Could you check a few things on this drawing? It's one solid part, dimensions in mm from its lowest x, y, z. Give positions to 0.01 mm unless a question says otherwise; leave off trailing zeros. Loops run counter-clockwise (first coordinate to the right, second up) from the corner with the lowest first, then second, coordinate; pieces in that order, holes last. Notation, with made-up numbers: M -36,35.25 L 9,35.25 A30 cw 9,59.25 Z; hole C -26.75,63.25 d11. An arc over 180 degrees is marked long. Answer as a JSON object with one key per item and string values.
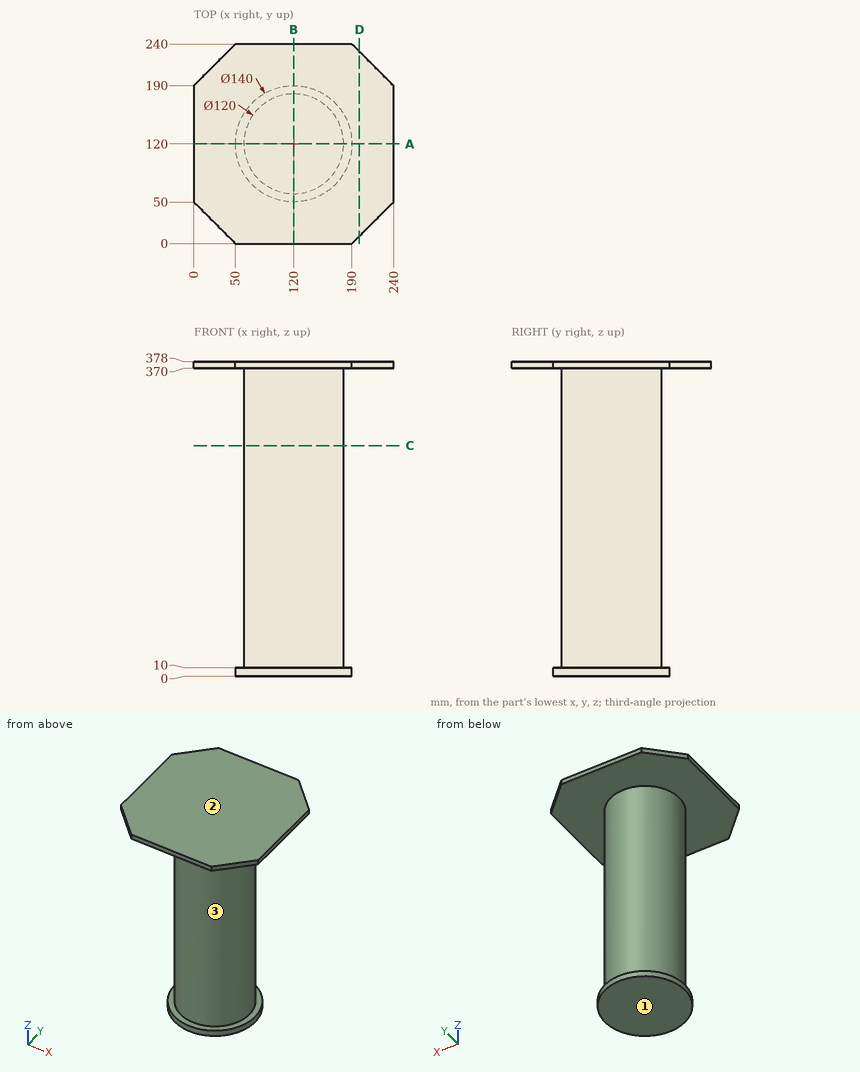
1) If we mould it in two halves opening along Z, with no side actions, what happens to the marked faces 1, 2 and 3? For each: +Z half, -Z half, draft (parallel to the pull), parting line (faces both ways), or undercut.
Answer list:
{"face 1": "-Z half", "face 2": "+Z half", "face 3": "undercut"}
2) Please list where these lines run through material, in increasing order: line 1 along Z through (x, y) = (79, 173.5); line 2 along Z through (x, y) = (205.5, 153.5); line 3 along Y through (x, z) = (119.5, 231). Write a range as from..to.
Answer list:
{"line 1": "0..10, 370..378", "line 2": "370..378", "line 3": "60..180"}
3) Will these pins go through, and if not, where does the flat tip stop? pin 1 Ø1.5 at (x, z) = (68, 68.5) entering from -Y; pin 2 Ø10 at (x, z) = (77.5, 195) entering from +Y; pin 3 Ø3 at (x, z) = (73, 141) entering from -Y.
Answer list:
{"pin 1": "y = 88.8", "pin 2": "y = 166.84", "pin 3": "y = 80.89"}
4) Suppose I cut it at D-D, the plane x = 199. Write out the boundary of the cut face in (y, z).
Answer list:
{"outline": "M 9,370 L 231,370 L 231,378 L 9,378 Z"}
5) Suppose I cut it at C-C, the plane z = 277. Write out the boundary of the cut face in (x, y).
Answer list:
{"outline": "C 120,120 d120"}
6) Suppose I cut it at A-A, the plane y = 120. Write out the boundary of the cut face in (x, z), and give its area (3 significant figures).
Answer list:
{"outline": "M 0,370 L 60,370 L 60,10 L 50,10 L 50,0 L 190,0 L 190,10 L 180,10 L 180,370 L 240,370 L 240,378 L 0,378 Z", "area": "46,500 mm^2"}
